Here's how the part is built. I have some questions about the finished solid (model axes, mm). Give positions to 0.01 mm unless a question says otherwise; leave off trailing zeros. Loops run counter-clockwise (first coordinate to the right, second up) from the corner with the lowest first, then second, coordinate; pieces in that order, holes last.
Q1. I'm going to push a flat-ended pin straight in: P1, Ø5, axis at x = 75.5, y = -14, coming from the -Z side. Where does the tip first touch, or does it pass through?
Q2. Suppose I cut it at B-B (x = 75). List the corners of the cut face in (y, z) for me, and give its area (3 significant figures).
Q3. Suppose I cut it at A-A (y = -30). List the corners of the cut face in (x, z) for me, and give its area (3 significant figures).
Q4. Suppose I cut it at C-C (z = 1.4). Count the separate pieces of the cut face and the enclosed holes in it, and give its area (3 significant figures).
Q5. I need wall thicknesses on probe 1 along Y at (x, z) = (52.5, 1.6); probe 2 along X at (y, z) = (47.5, 4.45); probe 3 along Y at (x, z) = (100.5, 1.35). Which ranges of each line are inside material? Lowest first, please.
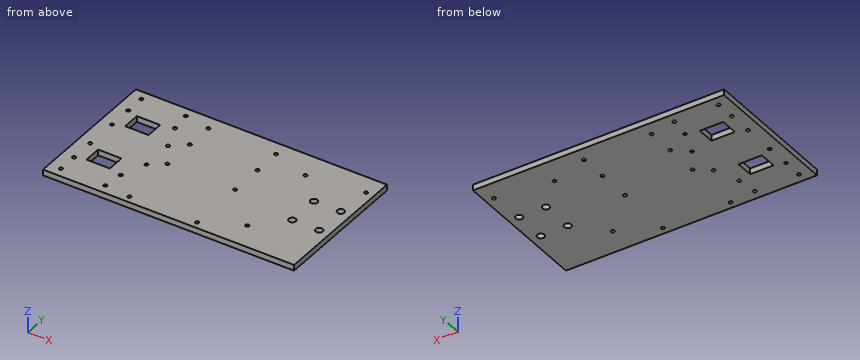
```python
from build123d import *

# Parameters (mm, degrees)
F0_W      = 215
F0_H      = 120
F1_DEPTH  = 5
F2_R      = 1.5
F2_W      = 20
F2_H      = 15
F3_DEPTH  = 25
F4_R      = 1.5
F5_DEPTH  = 5.001
F6_R      = 3
F7_DEPTH  = 5.001
F8_R      = 1.5
F9_DEPTH  = 5.001
F10_R     = 1.5
F11_DEPTH = 5.001
F12_R     = 1.5
F13_DEPTH = 5.001
F14_R     = 1.5
F15_DEPTH = 5.001


with BuildPart() as f1:
    # F0 (on Top) → F1 (new body)
    with BuildSketch(Plane.XY):
        Rectangle(F0_W, F0_H)
    extrude(amount=F1_DEPTH)

    # F2 (on face) → F3 (cut)
    with BuildSketch(Plane.XY.offset(5)):
        with Locations((-97.5, 52)):
            Circle(F2_R)
        with Locations((-59.5, 52)):
            Circle(F2_R)
        with Locations((-97.5, -52)):
            Circle(F2_R)
        with Locations((-59.5, -52)):
            Circle(F2_R)
        with Locations((-78.5, 25)):
            Rectangle(F2_W, F2_H)
        with Locations((-78.5, -25)):
            Rectangle(F2_W, F2_H)
    extrude(amount=-F3_DEPTH, mode=Mode.SUBTRACT)

    # F4 (on face) → F5 (cut, through all)
    with BuildSketch(Plane.XY.offset(5)):
        with Locations((-37.5, -54)):
            Circle(F4_R)
        with Locations((-37.5, -5)):
            Circle(F4_R)
        with Locations((20.5, -54)):
            Circle(F4_R)
        with Locations((20.5, -5)):
            Circle(F4_R)
    extrude(amount=-F5_DEPTH, mode=Mode.SUBTRACT)

    # F6 (on face) → F7 (cut, through all)
    with BuildSketch(Plane(origin=(0, 0, 0), x_dir=(1, 0, 0), z_dir=(0, 0, -1))):
        with Locations((98.5, -14)):
            Circle(F6_R)
        with Locations((98.5, 14)):
            Circle(F6_R)
        with Locations((75.5, -14)):
            Circle(F6_R)
        with Locations((75.5, 14)):
            Circle(F6_R)
    extrude(amount=-F7_DEPTH, mode=Mode.SUBTRACT)

    # F8 (on face) → F9 (cut, through all)
    with BuildSketch(Plane.XY.offset(5)):
        with Locations((-37.5, 48)):
            Circle(F8_R)
        with Locations((-37.5, 24)):
            Circle(F8_R)
        with Locations((20.5, 48)):
            Circle(F8_R)
        with Locations((20.5, 24)):
            Circle(F8_R)
    extrude(amount=-F9_DEPTH, mode=Mode.SUBTRACT)

    # F10 (on face) → F11 (cut, through all)
    with BuildSketch(Plane.XY.offset(5)):
        with Locations((-97.5, 14)):
            Circle(F10_R)
        with Locations((-97.5, -14)):
            Circle(F10_R)
        with Locations((-49.5, 14)):
            Circle(F10_R)
        with Locations((-49.5, -14)):
            Circle(F10_R)
    extrude(amount=-F11_DEPTH, mode=Mode.SUBTRACT)

    # F12 (on face) → F13 (cut, through all)
    with BuildSketch(Plane.XY.offset(5)):
        with Locations((-57.5, 35)):
            Circle(F12_R)
        with Locations((-57.5, -35)):
            Circle(F12_R)
        with Locations((-97.5, 35)):
            Circle(F12_R)
        with Locations((-97.5, -35)):
            Circle(F12_R)
    extrude(amount=-F13_DEPTH, mode=Mode.SUBTRACT)

    # F14 (on face) → F15 (cut, through all)
    with BuildSketch(Plane.XY.offset(5)):
        with Locations((52.5, 37.5)):
            Circle(F14_R)
        with Locations((100.5, 43.5)):
            Circle(F14_R)
        with Locations((52.5, -37.5)):
            Circle(F14_R)
    extrude(amount=-F15_DEPTH, mode=Mode.SUBTRACT)


solid = f1.part
```
Solutions:
1. P1: passes through
2. outline: (-60, 0) - (-16.96, 0) - (-16.96, 5) - (-60, 5) - close; (-11.04, 0) - (11.04, 0) - (11.04, 5) - (-11.04, 5) - close; (16.96, 0) - (60, 0) - (60, 5) - (16.96, 5) - close
2. area: 541 mm2
3. outline: (-107.5, 0) - (-88.5, 0) - (-88.5, 5) - (-107.5, 5) - close; (-68.5, 0) - (107.5, 0) - (107.5, 5) - (-68.5, 5) - close
3. area: 975 mm2
4. separate pieces: 1
4. enclosed holes: 29
4. area: 24,900 mm2
5. probe 1: y = -60 to -39, -36 to 36, 39 to 60
5. probe 2: x = -107.5 to -38.91, -36.09 to 19.09, 21.91 to 107.5
5. probe 3: y = -60 to -16.24, -11.76 to 11.76, 16.24 to 42, 45 to 60
